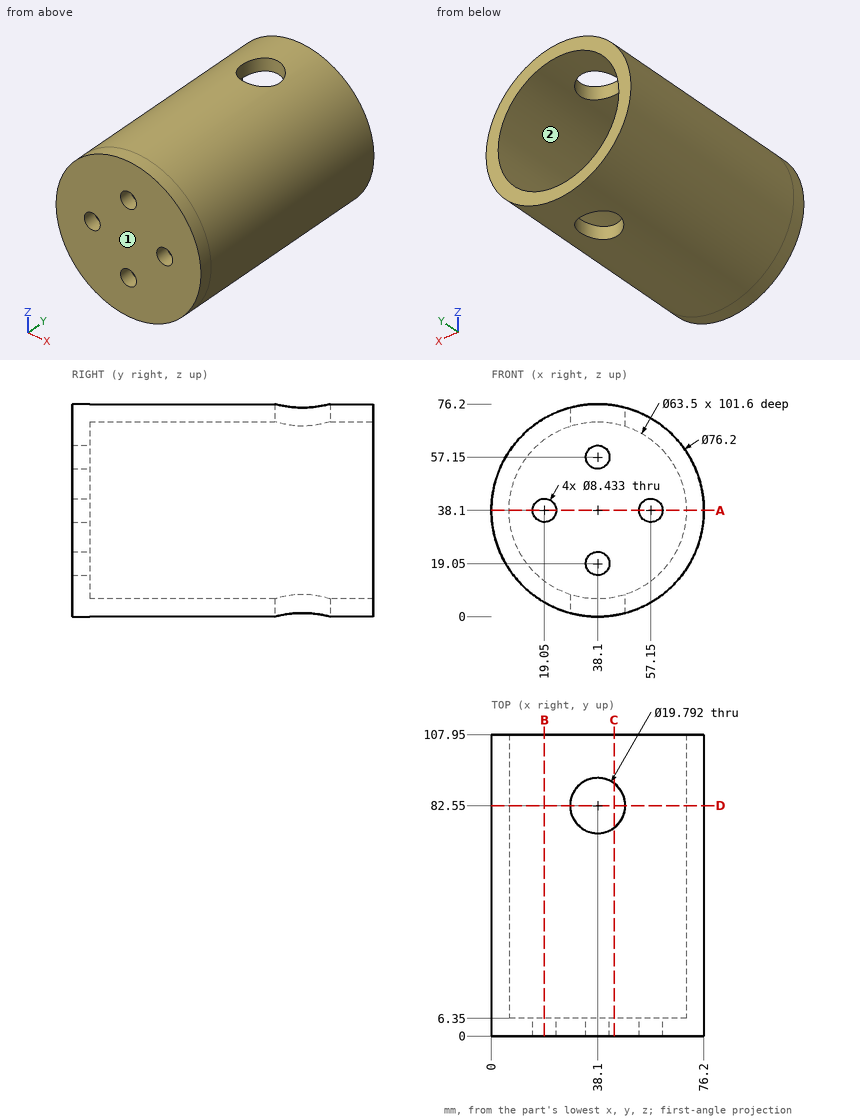
Could you check a few things on this drawing? It's one solid part, dimensions in mm from its lowest x, y, z. Round coordinates to 2 decimals unless told otherwise and drop trailing zeros. Write each loop counter-clockwise with the first axis right and the second up, starting at its lowest first coordinate (ties: lowest second). Pieces come first, ordered by that corner, then holes. Notation, with made-up numbers: M -22,-15.75 L 29,-15.75 A10 cw 29,0.25 Z; hole C -15.5,74 d2. An arc over 180 degrees is marked long. Answer as CSV lines item,"result". Start each with the question number.
1. Suppose I cut it at B-B on x = 19.05. Write out the boundary of the cut face in (y, z).
2. Suppose I cut it at D-D on y = 82.55. Write out the boundary of the cut face in (x, z).
3. Suppose I cut it at C-C on x = 44. Count the separate pieces of the cut face and the enclosed holes in it, then the cut area to 3 significant figures.
4. I need wall thicknesses on probe 1 along Z at (x, y) = (38, 2) (1 decimal); probe 2 along Y at (x, z) = (38, 3); probe 3 along Y at (x, z) = (32, 46.5). Which ranges of each line are inside material? Lowest first, please.
5. I'm going to push flat-ended pins straight in: pin 1 Ø9.5 at (x, z) = (57.15, 38.1) entering from +Y; pin 2 Ø2 at (x, y) = (17, 69.5) entering from -Z; pin 3 Ø10 at (y, z) = (63.5, 16) entering from +X. Where does each tip first touch, or does it pass through?
6. Suppose I cut it at A-A on z = 38.1. Write out the boundary of the cut face in (x, y), then the cut area to 3 significant figures.
7. Thinking about a two-plate mould opening in X: for the marked faces 1 and 2, which applies, released by +X, released by -X, zero draft, split by the parting line, or undercut?
Check result:
1,outline,"M 0,5.1 L 107.95,5.1 L 107.95,12.7 L 6.35,12.7 L 6.35,33.88 L 0,33.88 Z; M 0,42.32 L 6.35,42.32 L 6.35,63.5 L 107.95,63.5 L 107.95,71.1 L 0,71.1 Z"
2,outline,"M 28.2,1.31 L 28.2,7.93 A31.75 cw 28.2,68.27 L 28.2,74.89 A38.1 ccw Z; M 48,1.31 A38.1 ccw 48,74.89 L 48,68.27 A31.75 cw 48,7.93 Z"
3,separate pieces,"3"
3,enclosed holes,"0"
3,area,"1,580 mm2"
4,probe 1,"z = 0 to 14.8, 23.3 to 52.9, 61.4 to 76.2"
4,probe 2,"y = 0 to 72.65, 92.45 to 107.95"
4,probe 3,"y = 0 to 6.35"
5,pin 1,"stops at y = 6.35"
5,pin 2,"stops at z = 5.73"
5,pin 3,"stops at x = 72.15"
6,outline,"M 0,0 L 14.83,0 L 14.83,6.35 L 6.35,6.35 L 6.35,107.95 L 0,107.95 Z; M 23.27,0 L 52.93,0 L 52.93,6.35 L 23.27,6.35 Z; M 61.37,0 L 76.2,0 L 76.2,107.95 L 69.85,107.95 L 69.85,6.35 L 61.37,6.35 Z"
6,area,"1,670 mm2"
7,face 1,"zero draft"
7,face 2,"undercut"
